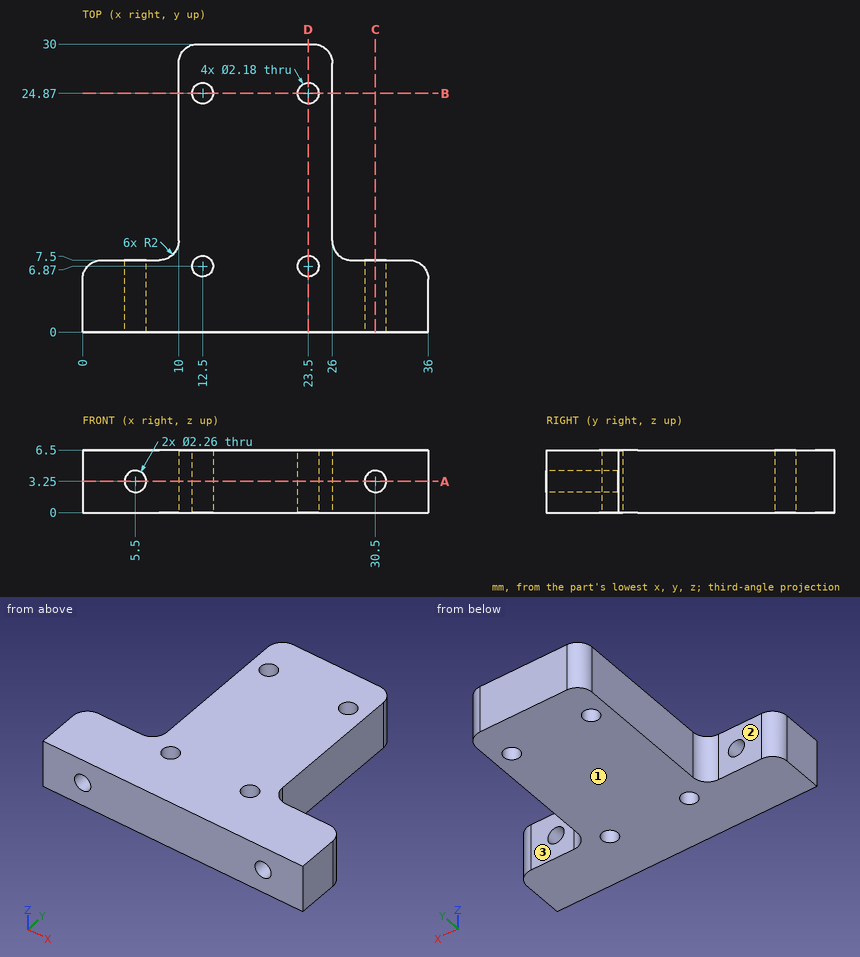
Here's the drawing with two shaded views (mm, measured from the low corner). I have some questions. A direction names the side the tool comes from. Give positions to 0.01 mm unless a question says otherwise; leave off trailing zeros. Write each loop counter-clockwise with the first axis right and the second up, starting at its lowest first coordinate (ties: lowest second). Pieces come first, ordered by that corner, then holes. Notation, with made-up numbers: (12.25, -40) - (67.25, -40) arc R19 cw to (67.25, -15) - close; hole circle Ø5 at (32.25, 55.5). An arc over 180 degrees is marked (long way). One line per item, written item: value. Start each with the question number.
Item 1: Imagine slicing it at A-A, the plane z = 3.25. List the corners of the cut face in (x, y) for me, and give its area (3 significant figures).
Item 2: Imagine slicing it at D-D, the plane x = 23.5. List the corners of the cut face in (y, z) for me.
Item 3: Imagine slicing it at C-C, the plane x = 30.5. List the corners of the cut face in (y, z) for me, and give its area (3 significant figures).
Item 4: I'm going to push flat-ended pins straight in: pin 1 (2 mm diameter, centred on y = 19, z = 2, fed in from -X); pin 2 (2 mm diameter, centred on y = 19, z = 3, fed in from +X); pin 3 (1.3 mm diameter, centred on x = 23.5, y = 24.87, fed in from -Z); pin 4 (3 mm diameter, centred on x = 31.5, z = 2, fed in from +Y). Where does each tip first touch, or does it pass through?
Item 5: Imagine slicing it at B-B, the plane y = 24.87. List the corners of the cut face in (x, z) for me.
Item 6: Please list where these lines run through material, in increasing order: line 1 (Y direction, x = 23.5, z = 3); line 2 (X direction, y = 24, z = 0.75); line 3 (Y direction, x = 13, z = 4). Write a range as from..to.
Item 7: Which directions (+Z, -Z, +X, -X, +Y, -Y) give clear straight access to the entire face, cutting with the end or side of a thin tool? Please do the marked faces 1, 2 and 3.
Geometry says:
1. outline: (0, 0) - (4.37, 0) - (4.37, 7.5) - (2, 7.5) arc R2 ccw to (0, 5.5) - close; (6.63, 0) - (29.37, 0) - (29.37, 7.5) - (28, 7.5) arc R2 cw to (26, 9.5) - (26, 28) arc R2 ccw to (24, 30) - (12, 30) arc R2 ccw to (10, 28) - (10, 9.5) arc R2 cw to (8, 7.5) - (6.63, 7.5) - close; (31.63, 0) - (36, 0) - (36, 5.5) arc R2 ccw to (34, 7.5) - (31.63, 7.5) - close; hole circle Ø2.18 at (12.5, 6.87); hole circle Ø2.18 at (12.5, 24.87); hole circle Ø2.18 at (23.5, 6.87); hole circle Ø2.18 at (23.5, 24.87)
1. area: 579 mm^2
2. outline: (0, 0) - (5.78, 0) - (5.78, 6.5) - (0, 6.5) - close; (7.96, 0) - (23.78, 0) - (23.78, 6.5) - (7.96, 6.5) - close; (25.96, 0) - (30, 0) - (30, 6.5) - (25.96, 6.5) - close
3. outline: (0, 0) - (7.5, 0) - (7.5, 2.12) - (0, 2.12) - close; (0, 4.38) - (7.5, 4.38) - (7.5, 6.5) - (0, 6.5) - close
3. area: 31.8 mm^2
4. pin 1: x = 10
4. pin 2: x = 26
4. pin 3: through
4. pin 4: y = 7.5
5. outline: (10, 0) - (11.41, 0) - (11.41, 6.5) - (10, 6.5) - close; (13.59, 0) - (22.41, 0) - (22.41, 6.5) - (13.59, 6.5) - close; (24.59, 0) - (26, 0) - (26, 6.5) - (24.59, 6.5) - close
6. line 1: 0..5.78, 7.96..23.78, 25.96..30
6. line 2: 10..11.84, 13.16..22.84, 24.16..26
6. line 3: 0..5.9, 7.84..23.9, 25.84..30
7. face 1: -Z, +X, -X, +Y, -Y
7. face 2: +Z, -Z, -X, +Y
7. face 3: +Z, -Z, +X, +Y
